Check sheet for the modelled part. Datum: model origin and axes. Units: mm. A direction names the side the tool comes from. Coordinates: 2 decimals unless noted, no trailing zeros. Loops run counter-clockwise (first coordinate to the right, second up) from the corner with the lowest first, then second, coordinate; pieces in that order, holes last. Notation, with made-up numbers: M 32.5,50 L 60.5,50 A20 ccw 60.5,67 Z; hole C -22,50.5 d11. An arc over 180 degrees is marked long. Use CSV: the item, a comma, the result in double quotes. Start each with the question number.
(1) Section check C-C on x = -11.5. Record the cut outline in (y, z), and give its area (3 significant figures).
(2) Scan lines: line 1 (X direction, y = 3.9, z = -72.5); line 2 (X direction, y = 0.55, z = -67.5); line 3 (Z direction, x = 57.5, y = 1.45). Record each from-to range of solid material in increasing order.
(3) Section check B-B on x = 23. Record the cut outline in (y, z).
(4) Go/stop test with flat-tipped pins: pin 1 Ø3 at (y, z) = (2, -11) entering from +X; pin 2 Ø1.8 at (x, y) = (28, 2) entering from -Z; pin 3 Ø3 at (x, y) = (-12.5, 1.5) entering from -Z. Record where each tip stops, or that it passes through.
(5) Set-up check for faces 5 (the flat face through (-114, 3, -105.84)), 6 (the cylindrical face through (50.65, 3.04, -31.58)), 7 (the flat face through (65, 3, -5)): record each of +Z, -Z, +X, -X, +Y, -Y from which the full face is reachable in a straight line by a thin tool's end or side.
(6) Section check A-A on y = 2.85. Give the number of separate pieces and of enclosed holes in the cut face, and give its area (3 significant figures).
(7) Draft check along X on faces 1 (the cylindrical face through (107.72, 3.04, -104.34)), 2 (the cylindrical face through (-119.8, 3, -104.4)), 3 (the cylindrical face through (64, 3, 13)), 4 (the flat face through (15, 3, -43)). Enter one of: pulls with the +X half, pulls with the -X half, needs draft (parallel to the pull), parting line crosses it, or undercut.
from build123d import *

# Parameters (mm, degrees)
BOSS_EXTRUDE1_DEPTH  = 6
FILLET1_R            = 5
SKETCH2_R            = 1.6
CUT_EXTRUDE1_DEPTH   = 162.089156951
FILLET1_OF_MIRROR1_R = 5


with BuildPart() as part:
    # Sketch1 → Boss-Extrude1 (new body)
    with BuildSketch(Plane(origin=(0, 0, 0), x_dir=(1, 0, 0), z_dir=(0, 1, 0))):
        Polygon((-50, 0), (-50, 32), (-106.291651246, 64.5), (-106.291651246, 105.839745962), (-121.291651246, 105.839745962), (-121.291651246, 55.839745962), (-65, 23.339745962), (-65, -15), (0, -15), (0, 0), (0, 80), (-15, 80), (-15, 0), align=None)
    boss_extrude1 = extrude(amount=BOSS_EXTRUDE1_DEPTH)

    # Fillet1
    fillet1_edges = [part.edges().sort_by_distance(p)[0] for p in [
        (-65, 3, 15),
        (-65, 3, -23.339745962),
        (-121.291651246, 3, -55.839745962),
        (-121.291651246, 3, -105.839745962),
        (-106.291651246, 3, -105.839745962),
        (-106.291651246, 3, -64.5),
        (-50, 3, -32),
        (-50, 3, 0),
        (-15, 3, 0),
    ]]
    fillet(fillet1_edges, radius=FILLET1_R)

    # Sketch2 → Cut-Extrude1 (cut, through all)
    with BuildSketch(Plane(origin=(0, 6, 0), x_dir=(1, 0, 0), z_dir=(0, 1, 0))):
        with Locations(Location((-7.5, 72.5, 0), (0, 0, 270))):
            Circle(SKETCH2_R)
        with Locations(Location((-57.5, 30, 0), (0, 0, 270))):
            Circle(SKETCH2_R)
        with Locations(Location((-57.5, 0, 0), (0, 0, 270))):
            Circle(SKETCH2_R)
    cut_extrude1 = extrude(amount=-CUT_EXTRUDE1_DEPTH, mode=Mode.SUBTRACT)

    # Mirror1: Boss-Extrude1, Cut-Extrude1 across plane
    add(boss_extrude1.mirror(Plane(origin=(0, 0, 0), x_dir=(0, 0, 1), z_dir=(1, 0, 0))))
    add(cut_extrude1.mirror(Plane(origin=(0, 0, 0), x_dir=(0, 0, 1), z_dir=(1, 0, 0))), mode=Mode.SUBTRACT)

    # Fillet1 of Mirror1
    fillet1_of_mirror1_edges = [part.edges().sort_by_distance(p)[0] for p in [
        (65, 3, 15),
        (65, 3, -23.339745962),
        (121.291651246, 3, -55.839745962),
        (121.291651246, 3, -105.839745962),
        (106.291651246, 3, -105.839745962),
        (106.291651246, 3, -64.5),
        (50, 3, -32),
        (50, 3, 0),
        (15, 3, 0),
    ]]
    fillet(fillet1_of_mirror1_edges, radius=FILLET1_OF_MIRROR1_R)


solid = part.part
Outcome:
1,outline,"M 0,-80 L 6,-80 L 6,15 L 0,15 Z"
1,area,"570 mm²"
2,line 1,"x = -121.29 to -106.29, -15 to -9.1, -5.9 to 5.9, 9.1 to 15, 106.29 to 121.29"
2,line 2,"x = -121.29 to -106.29, -15 to 15, 106.29 to 121.29"
2,line 3,"z = -36.33 to -31.6, -28.4 to -1.6, 1.6 to 15"
3,outline,"M 0,0 L 6,0 L 6,15 L 0,15 Z"
4,pin 1,"stops at x = 65"
4,pin 2,"stops at z = 0"
4,pin 3,"stops at z = -80"
5,face 5,"-Z, +X, -X, +Y, -Y"
5,face 6,"-Z, +Y, -Y"
5,face 7,"+Z, +X, +Y, -Y"
6,separate pieces,"1"
6,enclosed holes,"6"
6,area,"8,440 mm²"
7,face 1,"undercut"
7,face 2,"pulls with the -X half"
7,face 3,"pulls with the +X half"
7,face 4,"undercut"
